from build123d import *

# Parameters (mm, degrees)
SKETCH1_R           = 15
BOSS_EXTRUDE1_DEPTH = 30
SKETCH2_R           = 12
BOSS_EXTRUDE2_DEPTH = 5
SKETCH4_R           = 1.579295677
CUT_EXTRUDE3_DEPTH  = 3
SKETCH5_R           = 3
BOSS_EXTRUDE3_DEPTH = 40


with BuildPart() as part:
    # Sketch1 → Boss-Extrude1 (new body)
    with BuildSketch(Plane.XY):
        with Locations((5.178689325, -6.92509434)):
            Circle(SKETCH1_R)
    extrude(amount=BOSS_EXTRUDE1_DEPTH)

    # Sketch2 → Boss-Extrude2 (add)
    with BuildSketch(Plane.XY.offset(30)):
        with Locations((5.178689325, -6.92509434)):
            Circle(SKETCH2_R)
    extrude(amount=BOSS_EXTRUDE2_DEPTH)

    # Sketch4 → Cut-Extrude3 (cut)
    with BuildSketch(Plane.XY.offset(35)):
        with Locations((5.178689325, 2.995609984)):
            Circle(SKETCH4_R)
        with Locations((15.099393648, -6.92509434)):
            Circle(SKETCH4_R)
        with Locations((5.178689325, -16.845798663)):
            Circle(SKETCH4_R)
        with Locations((-4.742014998, -6.92509434)):
            Circle(SKETCH4_R)
    extrude(amount=-CUT_EXTRUDE3_DEPTH, mode=Mode.SUBTRACT)

    # Sketch5 → Boss-Extrude3 (add)
    with BuildSketch(Plane.XY.offset(35)):
        with Locations((5.178689325, -6.92509434)):
            Circle(SKETCH5_R)
    extrude(amount=BOSS_EXTRUDE3_DEPTH)


solid = part.part
Work out the finished part from the listing and answer in its coordinate system (mm). A direction names the side the tool comes from. Coordinates: 2 decimals unless noted, no trailing zeros. Order: outer loops, then holes, each group sorted by start corner. A loop starts at its lowest first (then second) coordinate and runs counter-clockwise, first axis right, second up. Notation, with made-up numbers: (55, -8) - (114, -8) arc R32 ccw to (114, 25) - close; hole circle Ø3 at (26, -38). An arc over 180 degrees is marked (long way). Put each result on its own line as item: value. Start each with the question number.
1) For faces 4 (the flat face through (5, 3, 32)), 5 (the cylindrical face through (19.035, -12.67, 14.79)), determine the directions among +Z, -Z, +X, -X, +Y, -Y from which every point of the face is accessible in a straight line to the end or side of a thin tool.
2) Find section D-D (y = -14.5). Give the vertices of the cut face in (x, z).
3) Find section C-C (z = 5). Give the vertices of the cut face in (x, y), plus the area to 3 significant figures.
4) Find the intervals of material crossed by line 1 (Z direction, x = 2.75, y = -13.25); line 2 (Z direction, x = 6.5, y = 6); line 3 (Y direction, x = 5.25, z = 72.5), in increasing order. Write a range as from..to.
5) Flat-ended cylindrical pins translate along their axes: pin 1 (4 mm diameter, centred on y = -14, z = 13, fed in from +X); pin 2 (3 mm diameter, centred on x = 15.1, y = -6.93, fed in from +Z); pin 3 (12 mm diameter, centred on y = -14, z = 32, fed in from -X). Find the tip coordinate at first contact, or state that the pin passes through.
6) For a pull along X with two mould halves and no side action, classify faces 1 (the flat face through (5, -7, 0)), 2 (the cylindrical face through (4.97, -15.28, 33.52)), 3 (the cylindrical face through (16.264, -11.521, 32.465)) as released by +X, released by -X, zero draft, split by the parting line, or undercut.
7) Find section A-A (y = -1). Give the vertices of the cut face in (x, z).
8) Find section B-B (x = -4.5). Give the vertices of the cut face in (y, z), plus the area to 3 significant figures.
Results list:
1. face 4: +Z
1. face 5: +Z, -Z
2. outline: (-7.77, 0) - (18.13, 0) - (18.13, 30) - (14.49, 30) - (14.49, 35) - (-4.13, 35) - (-4.13, 30) - (-7.77, 30) - close
3. outline: circle Ø30 at (5.18, -6.93)
3. area: 707 mm^2
4. line 1: z = 0..35
4. line 2: z = 0..30
4. line 3: y = -9.92..-3.93
5. pin 1: stops at x = 19.29
5. pin 2: stops at z = 32
5. pin 3: stops at x = -9.75
6. face 1: zero draft
6. face 2: undercut
6. face 3: split by the parting line
7. outline: (-8.6, 0) - (18.96, 0) - (18.96, 30) - (15.61, 30) - (15.61, 35) - (-5.26, 35) - (-5.26, 30) - (-8.6, 30) - close
8. outline: (-18.38, 0) - (4.53, 0) - (4.53, 30) - (0.17, 30) - (0.17, 35) - (-5.36, 35) - (-5.36, 32) - (-8.49, 32) - (-8.49, 35) - (-14.02, 35) - (-14.02, 30) - (-18.38, 30) - close
8. area: 749 mm^2
